from build123d import *

# Parameters (mm, degrees)
BOX056_W                = 72
BOX056_H                = 58
BOX056_DEPTH            = 4
BOX024_W                = 6
BOX024_H                = 36
BOX024_DEPTH            = 23
CYLINDER011_R           = 2.75
CYLINDER011_DEPTH       = 74.5
CYLINDER011_PITCH_ANGLE = 90
CYLINDER008_R           = 1.75
CYLINDER008_DEPTH       = 21.5
CYLINDER008_PITCH_ANGLE = 90
CYLINDER009_R           = 3
CYLINDER009_DEPTH       = 21.5
CYLINDER009_PITCH_ANGLE = 90
BOX007_W                = 3
BOX007_H                = 56
BOX007_DEPTH            = 6
BOX008_W                = 3
BOX008_H                = 56
BOX008_DEPTH            = 6
BOX006_W                = 4
BOX006_H                = 56
BOX006_DEPTH            = 21
CYLINDER003_R           = 1.75
CYLINDER003_DEPTH       = 74.5
CYLINDER003_PITCH_ANGLE = 90
BOX003_W                = 28
BOX003_H                = 88
BOX003_DEPTH            = 38
BOX002_W                = 28
BOX002_H                = 88
BOX002_DEPTH            = 38
BOX001_W                = 47
BOX001_H                = 42
BOX001_DEPTH            = 25
BOX_W                   = 72
BOX_H                   = 58
BOX_DEPTH               = 24
FILLET_R                = 10
CHAMFER_SIZE            = 3
CHAMFER110_1_SIZE       = 12
CHAMFER110_2_SIZE       = 7


with BuildPart() as cubo006:
    # Box056 → Box056 (new body)
    with BuildSketch(Plane(origin=(-15, -29, -2), x_dir=(1, 0, 0), z_dir=(0, 0, 1))):
        with Locations((36, 29)):
            Rectangle(BOX056_W, BOX056_H)
    extrude(amount=BOX056_DEPTH)


with BuildPart() as cube024:
    # Box024 → Box024 (new body)
    with BuildSketch(Plane(origin=(0, 19, 7), x_dir=(1, 0, 0), z_dir=(0, 0, 1))):
        with Locations((3, 18)):
            Rectangle(BOX024_W, BOX024_H)
    extrude(amount=BOX024_DEPTH)


with BuildPart() as joint_d013:
    # Cylinder011 → Cylinder011 (new body)
    with BuildSketch(Plane.XY):
        Circle(CYLINDER011_R)
    extrude(amount=CYLINDER011_DEPTH)


with BuildPart() as joint_d013_1:
    # Cylinder011 pitch: moved
    add(joint_d013.part.rotate(Axis((0, 0, 0), (0, 1, 0)), CYLINDER011_PITCH_ANGLE))


with BuildPart() as joint_d013_2:
    # Cylinder011 placement: moved
    add(joint_d013_1.part.moved(Location((-3, 9.5, 12))))


with BuildPart() as joint_d010:
    # Cylinder008 → Cylinder008 (new body)
    with BuildSketch(Plane.XY):
        Circle(CYLINDER008_R)
    extrude(amount=CYLINDER008_DEPTH)


with BuildPart() as joint_d010_1:
    # Cylinder008 pitch: moved
    add(joint_d010.part.rotate(Axis((0, 0, 0), (0, 1, 0)), CYLINDER008_PITCH_ANGLE))


with BuildPart() as joint_d010_2:
    # Cylinder008 placement: moved
    add(joint_d010_1.part.moved(Location((16, -24.5, 7))))


with BuildPart() as joint_d011:
    # Cylinder009 → Cylinder009 (new body)
    with BuildSketch(Plane.XY):
        Circle(CYLINDER009_R)
    extrude(amount=CYLINDER009_DEPTH)


with BuildPart() as joint_d011_1:
    # Cylinder009 pitch: moved
    add(joint_d011.part.rotate(Axis((0, 0, 0), (0, 1, 0)), CYLINDER009_PITCH_ANGLE))


with BuildPart() as joint_d011_2:
    # Cylinder009 placement: moved
    add(joint_d011_1.part.moved(Location((32, -24.5, 7))))


with BuildPart() as fusion001:
    # Fusion001 base: copy of Joint-D011
    add(joint_d011_2.part)

    # Fusion001: union Joint-D010
    add(joint_d010_2.part)


with BuildPart() as fusion002:
    # Fusion002 base: copy of Joint-D011
    add(joint_d011_2.part)

    # Fusion002: union Joint-D010
    add(joint_d010_2.part)


with BuildPart() as fusion002_1:
    # Fusion002 placement: moved
    add(fusion002.part.moved(Location((0, 0, 10))))


with BuildPart() as fusion003:
    # Fusion003 base: copy of Joint-D011
    add(joint_d011_2.part)

    # Fusion003: union Joint-D010
    add(joint_d010_2.part)


with BuildPart() as fusion003_1:
    # Fusion003 placement: moved
    add(fusion003.part.moved(Location((0, 49, 0))))


with BuildPart() as fusion004:
    # Fusion004 base: copy of Joint-D011
    add(joint_d011_2.part)

    # Fusion004: union Joint-D010
    add(joint_d010_2.part)


with BuildPart() as fusion004_1:
    # Fusion004 placement: moved
    add(fusion004.part.moved(Location((0, 49, 10))))


with BuildPart() as cube007:
    # Box007 → Box007 (new body)
    with BuildSketch(Plane(origin=(18.5, -28, 4), x_dir=(1, 0, 0), z_dir=(0, 0, 1))):
        with Locations((1.5, 28)):
            Rectangle(BOX007_W, BOX007_H)
    extrude(amount=BOX007_DEPTH)


with BuildPart() as cube008:
    # Box008 → Box008 (new body)
    with BuildSketch(Plane(origin=(18.5, -28, 14), x_dir=(1, 0, 0), z_dir=(0, 0, 1))):
        with Locations((1.5, 28)):
            Rectangle(BOX008_W, BOX008_H)
    extrude(amount=BOX008_DEPTH)


with BuildPart() as cube006:
    # Box006 → Box006 (new body)
    with BuildSketch(Plane(origin=(25.5, -28, 2), x_dir=(1, 0, 0), z_dir=(0, 0, 1))):
        with Locations((2, 28)):
            Rectangle(BOX006_W, BOX006_H)
    extrude(amount=BOX006_DEPTH)


with BuildPart() as joint_d005:
    # Cylinder003 → Cylinder003 (new body)
    with BuildSketch(Plane.XY):
        Circle(CYLINDER003_R)
    extrude(amount=CYLINDER003_DEPTH)


with BuildPart() as joint_d005_1:
    # Cylinder003 pitch: moved
    add(joint_d005.part.rotate(Axis((0, 0, 0), (0, 1, 0)), CYLINDER003_PITCH_ANGLE))


with BuildPart() as joint_d005_2:
    # Cylinder003 placement: moved
    add(joint_d005_1.part.moved(Location((-22, 9.5, 12))))


with BuildPart() as cube003:
    # Box003 → Box003 (new body)
    with BuildSketch(Plane(origin=(-33, -45, 1), x_dir=(1, 0, 0), z_dir=(0, 0, 1))):
        with Locations((14, 44)):
            Rectangle(BOX003_W, BOX003_H)
    extrude(amount=BOX003_DEPTH)


with BuildPart() as cube002:
    # Box002 → Box002 (new body)
    with BuildSketch(Plane(origin=(37, -45, 1), x_dir=(1, 0, 0), z_dir=(0, 0, 1))):
        with Locations((14, 44)):
            Rectangle(BOX002_W, BOX002_H)
    extrude(amount=BOX002_DEPTH)


with BuildPart() as cube001:
    # Box001 → Box001 (new body)
    with BuildSketch(Plane(origin=(-1, -21, 2), x_dir=(1, 0, 0), z_dir=(0, 0, 1))):
        with Locations((23.5, 21)):
            Rectangle(BOX001_W, BOX001_H)
    extrude(amount=BOX001_DEPTH)


with BuildPart() as obj1:
    # Box → Box (new body)
    with BuildSketch(Plane(origin=(-15, -29, -3), x_dir=(1, 0, 0), z_dir=(0, 0, 1))):
        with Locations((36, 29)):
            Rectangle(BOX_W, BOX_H)
    extrude(amount=BOX_DEPTH)

    # Cut: cut Cube001
    add(cube001.part, mode=Mode.SUBTRACT)

    # Cut001: cut Cube002
    add(cube002.part, mode=Mode.SUBTRACT)

    # Cut002: cut Cube003
    add(cube003.part, mode=Mode.SUBTRACT)

    # Fillet
    fillet_edges = [obj1.edges().sort_by_distance(p)[0] for p in [
        (-15, -29, -1),
        (-15, 29, -1),
        (57, -29, -1),
        (57, 29, -1),
    ]]
    fillet(fillet_edges, radius=FILLET_R)

    # Chamfer
    chamfer_edges = [obj1.edges().sort_by_distance(p)[0] for p in [
        (-5, 0, 21),
        (37, 25, 21),
        (37, -25, 21),
    ]]
    chamfer(chamfer_edges, length=CHAMFER_SIZE)

    # Cut008: cut Joint-D005
    add(joint_d005_2.part, mode=Mode.SUBTRACT)

    # Cut010: cut Cube006
    add(cube006.part, mode=Mode.SUBTRACT)

    # Cut011: cut Cube008
    add(cube008.part, mode=Mode.SUBTRACT)

    # Cut012: cut Cube007
    add(cube007.part, mode=Mode.SUBTRACT)

    # Cut013: cut Fusion004
    add(fusion004_1.part, mode=Mode.SUBTRACT)

    # Cut014: cut Fusion003
    add(fusion003_1.part, mode=Mode.SUBTRACT)

    # Cut015: cut Fusion002
    add(fusion002_1.part, mode=Mode.SUBTRACT)

    # Cut016: cut Fusion001
    add(fusion001.part, mode=Mode.SUBTRACT)

    # Cut017: cut Joint-D013
    add(joint_d013_2.part, mode=Mode.SUBTRACT)

    # Cut039: cut Cube024
    add(cube024.part, mode=Mode.SUBTRACT)


with BuildPart() as obj1_1:
    # Cut039 placement: moved
    add(obj1.part.moved(Location((0, 0, 1))))

    # Fusion060: union Cubo006
    add(cubo006.part)

    # Chamfer110 1
    chamfer110_1_edges = [obj1_1.edges().sort_by_distance(p)[0] for p in [
        (57, -29, 0),
    ]]
    chamfer(chamfer110_1_edges, length=CHAMFER110_1_SIZE)

    # Chamfer110 2
    chamfer110_2_edges = [obj1_1.edges().sort_by_distance(p)[0] for p in [
        (-15, -29, 0),
        (57, 29, 0),
        (-15, 29, 0),
    ]]
    chamfer(chamfer110_2_edges, length=CHAMFER110_2_SIZE)


solid = obj1_1.part
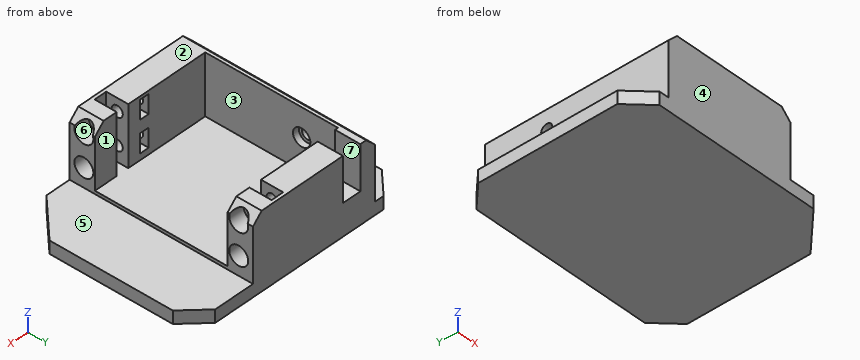
Input: part model. Units: mm. Frame: model coordinates. Face numbers are marked on the shaded views. A direction names the side the tool comes from. Round coordinates to 2 decimals unless told otherwise and drop trailing zeros. Write each loop counter-clockwise with the first axis right and the second up, starting at its lowest first coordinate (ties: lowest second). Pieces come first, ordered by that corner, then holes.
1) Contact query for flat-ended pins moving along their axis: P1, Ø4, axis at y = -17, z = 7.5, coming from the -X side; P2, Ø5.5, axis at y = 24.5, z = 8, coming from the +X side; P3, Ø3, axis at x = 4, z = 17, coming from the +Y side. Output: stop coordinate, or through.
2) Cut plane D-D (z = 18). Count the separate pieces of the cut face and the enclosed holes in it, then the cut area to 3 significant figures.
3) Cut plane B-B (z = 13). Return the cut outline in (x, y), then the cut area to 3 significant figures.
4) Cut plane A-A (y = 9.5). Return the cut outline in (x, z).
5) Ray query, L1, parallel to Y at x = 34.4, z = 18; L2, parallel to Y at x = 23.55, z = 18; L3, parallel to Z at x = 22.7, y = -24.5. Return the intervals inside material, ascending.
6) Reachability of the marked faces 5, 6 and 7 from +Z, -Z, +X, -X, +Y, -Y: full face, straight path, thin tool, end or side. Return the list, or none.
7) Draft query along Y for the marked faces 1, 2, 3 and 4. Return one class per face: pulls with the +Y half, pulls with the -Y half, needs draft (parallel to the pull), parting line crosses it, or undercut.
8) Cut plane C-C (x = 2.5). Return the cut outline in (y, z).
Geometry says:
1. P1: stops at x = -5
1. P2: stops at x = 32
1. P3: stops at y = -21
2. separate pieces: 6
2. enclosed holes: 0
2. area: 571 mm2
3. outline: (-5, -29) - (37, -29) - (37, -21) - (29.5, -21) - (29.5, -28) - (25.5, -28) - (25.5, -21) - (-1, -21) - (-1, 6.75) - (-3, 6.75) - (-3, 7.75) - (-5, 7.75) - close; (-5, 11.25) - (-3, 11.25) - (-3, 12.25) - (-1, 12.25) - (-1, 21) - (0, 21) - (0, 29) - (-5, 29) - close; (6, 21) - (25.5, 21) - (25.5, 28) - (29.5, 28) - (29.5, 21) - (37, 21) - (37, 29) - (6, 29) - close
3. area: 718 mm2
4. outline: (-15, -2) - (57, -2) - (57, 2) - (37, 2) - (37, 3) - (-1, 3) - (-1, 10.25) - (-3, 10.25) - (-3, 11.25) - (-5, 11.25) - (-5, 2) - (-15, 2) - close; (-5, 14.75) - (-3, 14.75) - (-3, 15.75) - (-1, 15.75) - (-1, 22) - (-2, 22) - (-5, 19) - close
5. L1: y = -29 to -27.5, -21.5 to -21, 21 to 21.5, 27.5 to 29
5. L2: y = -29 to -26.25, -22.75 to -21, 21 to 22.75, 26.25 to 29
5. L3: z = -2 to 6.25, 9.75 to 16.25, 19.75 to 22
6. face 5: +Z, +X, +Y, -Y
6. face 6: +X
6. face 7: +Z, +Y
7. face 1: undercut
7. face 2: needs draft
7. face 3: undercut
7. face 4: pulls with the -Y half
8. outline: (-29, -2) - (29, -2) - (29, 8) - (21, 8) - (21, 3) - (-21, 3) - (-21, 22) - (-29, 22) - close
